Geometry check sheet. Reference: the model listing, model coordinates, mm. A direction names the side the tool comes from. Coordinates: 2 decimals unless noted, no trailing zeros. Loops run counter-clockwise (first coordinate to the right, second up) from the corner with the lowest first, then second, coordinate; pieces in that order, holes last. Notation, with made-up numbers: (-14.5, 77) -> (4.5, 77) arc R6 ccw to (4.5, 82) -> close; hole circle Ø7 at (-13, 49). An arc over 180 degrees is marked (long way). Answer as a JSON object with one key per item and string values.
from build123d import *

# Parameters (mm, degrees)
BOSS_EXTRUDE1_DEPTH   = 255.5875
BOSS_EXTRUDE1_2_DEPTH = 255.5875
BOSS_EXTRUDE1_3_DEPTH = 255.5875
SKETCH4_W             = 120.65
SKETCH4_H             = 19.812
BOSS_EXTRUDE2_DEPTH   = 255.5875
SKETCH5_R             = 1.524
BOSS_EXTRUDE3_DEPTH   = 511.175
SKETCH_PATTERN1_START = -255.5875
SKETCH_PATTERN1_DEPTH = 511.175
BOSS_EXTRUDE4_DEPTH   = 304.8


# Read off the part's stored shape, not the designer's step: Sketch-Pattern1
with BuildPart() as part:
    # Sketch3 → Boss-Extrude1 (new, symmetric)
    with BuildSketch(Plane.XY):
        Polygon((-304.8, -76.2), (-304.8, -73.025), (-287.655, -55.5625), (-201.295, -55.5625), (-184.15, -73.025), (-184.15, -76.2), align=None)
    extrude(amount=BOSS_EXTRUDE1_DEPTH, both=True)



with BuildPart() as body_2:
    # Sketch3 → Boss-Extrude1 2 (new, symmetric)
    with BuildSketch(Plane.XY):
        Polygon((184.15, -73.025), (184.15, -76.2), (304.8, -76.2), (304.8, -73.025), (287.655, -55.5625), (201.295, -55.5625), align=None)
    extrude(amount=BOSS_EXTRUDE1_2_DEPTH, both=True)


with BuildPart() as body_3:
    # Sketch3 → Boss-Extrude1 3 (new, symmetric)
    with BuildSketch(Plane.XY):
        Polygon((-43.18, -55.5625), (43.18, -55.5625), (60.325, -73.025), (60.325, -76.2), (-60.325, -76.2), (-60.325, -73.025), align=None)
    extrude(amount=BOSS_EXTRUDE1_3_DEPTH, both=True)


with BuildPart() as body_4:
    # Sketch4 → Boss-Extrude2 (new, symmetric)
    with BuildSketch(Plane.XY):
        with Locations((-244.475, 63.881)):
            Rectangle(SKETCH4_W, SKETCH4_H)
    extrude(amount=BOSS_EXTRUDE2_DEPTH, both=True)

    # Sketch5 → Boss-Extrude3 (add)
    with BuildSketch(Plane.XY.offset(255.5875)):
        with Locations((-294.005, 72.644)):
            Circle(SKETCH5_R)
        with Locations((-284.099, 72.644)):
            Circle(SKETCH5_R)
        with Locations((-274.193, 72.644)):
            Circle(SKETCH5_R)
        with Locations((-264.287, 72.644)):
            Circle(SKETCH5_R)
        with Locations((-254.381, 72.644)):
            Circle(SKETCH5_R)
        with Locations((-244.475, 72.644)):
            Circle(SKETCH5_R)
        with Locations((-234.569, 72.644)):
            Circle(SKETCH5_R)
        with Locations((-224.663, 72.644)):
            Circle(SKETCH5_R)
        with Locations((-214.757, 72.644)):
            Circle(SKETCH5_R)
        with Locations((-204.851, 72.644)):
            Circle(SKETCH5_R)
    extrude(amount=-BOSS_EXTRUDE3_DEPTH)


with BuildPart() as body_5:
    # Sketch-Pattern1 outline → Sketch-Pattern1 (new body)
    with BuildSketch(Plane.XY.offset(SKETCH_PATTERN1_START)):
        with BuildLine():
            Line((60.325, 73.787), (40.63203125, 73.787))
            ThreePointArc((40.63203125, 73.787), (39.624, 74.168), (38.61596875, 73.787))
            Line((38.61596875, 73.787), (30.72603125, 73.787))
            ThreePointArc((30.72603125, 73.787), (29.718, 74.168), (28.70996875, 73.787))
            Line((28.70996875, 73.787), (20.82003125, 73.787))
            ThreePointArc((20.82003125, 73.787), (19.812, 74.168), (18.80396875, 73.787))
            Line((18.80396875, 73.787), (10.91403125, 73.787))
            ThreePointArc((10.91403125, 73.787), (9.906, 74.168), (8.89796875, 73.787))
            Line((8.89796875, 73.787), (1.00803125, 73.787))
            ThreePointArc((1.00803125, 73.787), (0, 74.168), (-1.00803125, 73.787))
            Line((-1.00803125, 73.787), (-8.89796875, 73.787))
            ThreePointArc((-8.89796875, 73.787), (-9.906, 74.168), (-10.91403125, 73.787))
            Line((-10.91403125, 73.787), (-18.80396875, 73.787))
            ThreePointArc((-18.80396875, 73.787), (-19.812, 74.168), (-20.82003125, 73.787))
            Line((-20.82003125, 73.787), (-28.70996875, 73.787))
            ThreePointArc((-28.70996875, 73.787), (-29.718, 74.168), (-30.72603125, 73.787))
            Line((-30.72603125, 73.787), (-38.61596875, 73.787))
            ThreePointArc((-38.61596875, 73.787), (-39.624, 74.168), (-40.63203125, 73.787))
            Line((-40.63203125, 73.787), (-48.52196875, 73.787))
            ThreePointArc((-48.52196875, 73.787), (-49.53, 74.168), (-50.53803125, 73.787))
            Line((-50.53803125, 73.787), (-60.325, 73.787))
            Line((-60.325, 73.787), (-60.325, 53.975))
            Line((-60.325, 53.975), (60.325, 53.975))
            Line((60.325, 53.975), (60.325, 73.787))
        make_face()
        with BuildLine():
            Line((304.8, 73.787), (285.10703125, 73.787))
            ThreePointArc((285.10703125, 73.787), (284.099, 74.168), (283.09096875, 73.787))
            Line((283.09096875, 73.787), (275.20103125, 73.787))
            ThreePointArc((275.20103125, 73.787), (274.193, 74.168), (273.18496875, 73.787))
            Line((273.18496875, 73.787), (265.29503125, 73.787))
            ThreePointArc((265.29503125, 73.787), (264.287, 74.168), (263.27896875, 73.787))
            Line((263.27896875, 73.787), (255.38903125, 73.787))
            ThreePointArc((255.38903125, 73.787), (254.381, 74.168), (253.37296875, 73.787))
            Line((253.37296875, 73.787), (245.48303125, 73.787))
            ThreePointArc((245.48303125, 73.787), (244.475, 74.168), (243.46696875, 73.787))
            Line((243.46696875, 73.787), (235.57703125, 73.787))
            ThreePointArc((235.57703125, 73.787), (234.569, 74.168), (233.56096875, 73.787))
            Line((233.56096875, 73.787), (225.67103125, 73.787))
            ThreePointArc((225.67103125, 73.787), (224.663, 74.168), (223.65496875, 73.787))
            Line((223.65496875, 73.787), (215.76503125, 73.787))
            ThreePointArc((215.76503125, 73.787), (214.757, 74.168), (213.74896875, 73.787))
            Line((213.74896875, 73.787), (205.85903125, 73.787))
            ThreePointArc((205.85903125, 73.787), (204.851, 74.168), (203.84296875, 73.787))
            Line((203.84296875, 73.787), (195.95303125, 73.787))
            ThreePointArc((195.95303125, 73.787), (194.945, 74.168), (193.93696875, 73.787))
            Line((193.93696875, 73.787), (184.15, 73.787))
            Line((184.15, 73.787), (184.15, 53.975))
            Line((184.15, 53.975), (304.8, 53.975))
            Line((304.8, 53.975), (304.8, 73.787))
        make_face()
    extrude(amount=SKETCH_PATTERN1_DEPTH)


with BuildPart() as part_1:
    add(part.part)

    add(body_2.part)  # Boss-Extrude4 merges body 2

    add(body_3.part)  # Boss-Extrude4 merges body 3

    add(body_4.part)  # Boss-Extrude4 merges body 4

    add(body_5.part)  # Boss-Extrude4 merges body 5
    # Sketch8 → Boss-Extrude4 (add, symmetric)
    with BuildSketch(Plane(origin=(0, 0, 0), x_dir=(0, 0, -1), z_dir=(1, 0, 0))):
        Polygon((-255.5875, -76.2), (-255.5875, -50.3809), (-233.2355, -50.3809), (-233.2355, 50.927), (-255.5875, 50.927), (-255.5875, 76.2), (-252.5395, 76.2), (-252.5395, 53.975), (-230.1875, 53.975), (-230.1875, -53.4289), (-252.5395, -53.4289), (-252.5395, -76.2), align=None)
        Polygon((252.5395, -53.4289), (252.5395, -76.2), (255.5875, -76.2), (255.5875, -50.3809), (233.2355, -50.3809), (233.2355, 50.927), (255.5875, 50.927), (255.5875, 76.2), (252.5395, 76.2), (252.5395, 53.975), (230.1875, 53.975), (230.1875, -53.4289), align=None)
    extrude(amount=BOSS_EXTRUDE4_DEPTH, both=True)


solid = part_1.part
1. Mould release check, pull along X, two halves, no side actions. Record for faces 1 (the face through (296.35, -64.42, 3.54)), 2 (the face through (-121, 53.975, -242)), 3 (the face through (4, -50.381, -245)): released by +X, released by -X, zero draft, split by the parting line, or undercut.
Evaluation:
{"face 1": "released by +X", "face 2": "undercut", "face 3": "zero draft"}
2. Thickness scan on probe 1 along Z at (x, y) = (-184.5, -61); probe 2 along Z at (x, y) = (257.5, 3.5); probe 3 along Y at (x, z) = (-39.5, -3.5) (1 decimal). Record the ranges inside material, lowest first. Write a range as from..to.
Evaluation:
{"probe 1": "z = -255.59..-252.54, 252.54..255.59", "probe 2": "z = -233.24..-230.19, 230.19..233.24", "probe 3": "y = -76.2..-55.6, 54..74.2"}
3. Section check B-B, the plane x = 88. Record the boundary of the cut face in (y, z) (1 decimal), then the cut area to 3 significant figures.
Evaluation:
{"outline": "(-76.2, -255.6) -> (-50.4, -255.6) -> (-50.4, -233.2) -> (50.9, -233.2) -> (50.9, -255.6) -> (76.2, -255.6) -> (76.2, -252.5) -> (54, -252.5) -> (54, -230.2) -> (-53.4, -230.2) -> (-53.4, -252.5) -> (-76.2, -252.5) -> close; (-76.2, 252.5) -> (-53.4, 252.5) -> (-53.4, 230.2) -> (54, 230.2) -> (54, 252.5) -> (76.2, 252.5) -> (76.2, 255.6) -> (50.9, 255.6) -> (50.9, 233.2) -> (-50.4, 233.2) -> (-50.4, 255.6) -> (-76.2, 255.6) -> close", "area": "1,200 mm^2"}
4. Section check A-A, the plane y = -1. Record the boundary of the cut face in (x, z), then the cut area to 3 significant figures.
Evaluation:
{"outline": "(-304.8, -233.24) -> (304.8, -233.24) -> (304.8, -230.19) -> (-304.8, -230.19) -> close; (-304.8, 230.19) -> (304.8, 230.19) -> (304.8, 233.24) -> (-304.8, 233.24) -> close", "area": "3,720 mm^2"}
5. Section check C-C, the plane z = 24.5. State how many separate pieces and enclosed holes the cut face has, then the cut area to 3 significant figures.
Evaluation:
{"separate pieces": "6", "enclosed holes": "0", "area": "13,800 mm^2"}
6. Tool access check on faces 4 (the face through (245, -55.562, 4)), 5 (the face through (-192.843, -64.172, 3.536)), 6 (the face through (-4, 0, 233.236)), 7 (the face through (-123, 53.975, 242)). Record the directions out of +Z, -Z, +X, -X, +Y, -Y that give a thin tool (end or side, any length) a straight path to the whole face; none if there is none.
Evaluation:
{"face 4": "+X, -X", "face 5": "none", "face 6": "+Z, +X, -X", "face 7": "+Y"}
7. Depth check by flat-ended pin: P1, Ø6.5, axis at x = 35, z = -70, coming from the +Y side; P2, Ø2, axis at x = -51, y = -17, coming from the +Z side; P3, Ø8.5, axis at x = -33.5, z = -99.5, coming from the +Y side. Enter the tip coordinate at first touch or a pass-through.
Evaluation:
{"P1": "stops at y = 73.79", "P2": "stops at z = 233.24", "P3": "stops at y = 74.17"}
